from build123d import *

# Parameters (mm, degrees)
F0_R     = 1.5
F0_R_2   = 1.2
F0_R_3   = 1
F1_DEPTH = 85
F2_DEPTH = 2.5
F3_DEPTH = 4
F4_R     = 1
F6_START = -1
F5_W     = 21.3047601283
F5_H     = 75
F6_DEPTH = 1


with BuildPart() as f1:
    # F0 (on Top) → F1 (new body)
    with BuildSketch(Plane.XY):
        Circle(F0_R)
        Circle(F0_R_2, mode=Mode.SUBTRACT)
        Circle(F0_R_2)
        Circle(F0_R_3, mode=Mode.SUBTRACT)
        Circle(F0_R_3)
    extrude(amount=F1_DEPTH)

    # F0 (on Top) → F2 (cut)
    with BuildSketch(Plane.XY):
        Circle(F0_R)
        Circle(F0_R_2, mode=Mode.SUBTRACT)
    extrude(amount=F2_DEPTH, mode=Mode.SUBTRACT)

    # F0 (on Top) → F3 (cut)
    with BuildSketch(Plane.XY):
        Circle(F0_R_3)
    extrude(amount=F3_DEPTH, mode=Mode.SUBTRACT)

    # F4
    f4_edges = [f1.edges().sort_by_distance(p)[0] for p in [
        (-1.5, 0, 85),
    ]]
    fillet(f4_edges, radius=F4_R)

    # F5 (on Front) → F6 (join)
    with BuildSketch(Plane.XZ.offset(F6_START)):
        with Locations((10.6523800641, 40)):
            Rectangle(F5_W, F5_H)
    extrude(amount=-F6_DEPTH)


solid = f1.part
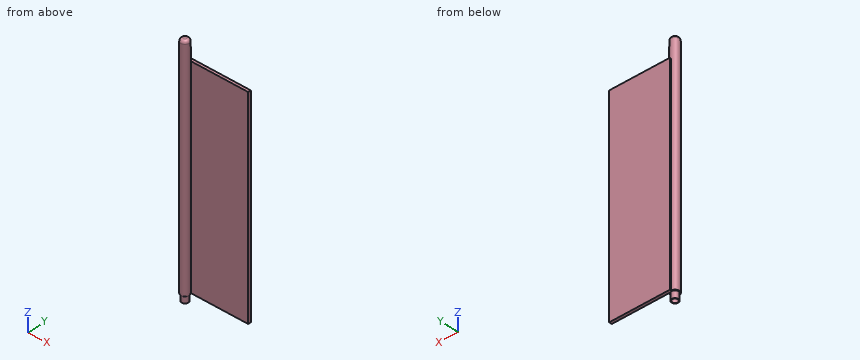
Geometry: final body of the model. Coordinates: model frame, mm. Give positions to 0.01 mm unless a question says otherwise; leave off trailing zeros. Order: outer loops, then holes, each group sorted by start corner. A loop starts at its lowest first (then second) coordinate and runs counter-clockwise, first axis right, second up. Notation, with made-up numbers: (19.25, 8.5) -> (65.25, 8.5) arc R26 cw to (65.25, 33.5) -> close; hole circle Ø7 at (-8.75, -10). An arc over 180 degrees is marked (long way). Answer as a JSON object with one key per item and string values.
Q1. First-contact query: pin 1 (0.8 mm diameter, centred on x = 6.5, y = 1.5, fed in from +Z); pin 2 (1.5 mm diameter, centred on x = 3, z = 69, fed in from -Y); pin 3 (1 mm diameter, centred on x = 9.5, y = 1, fed in from -Z); pin 4 (1 mm diameter, centred on x = 0.5, y = -0.5, fed in from -Z). Flat tips, straight axial feed; report the tip coordinate or a pass-through.
Entries:
{"pin 1": "stops at z = 77.5", "pin 2": "stops at y = 1", "pin 3": "stops at z = 2.5", "pin 4": "stops at z = 0"}
Q2. Section A-A (z = 12.5). Output: boundary loops of the cut face in (x, y), plus the area to 3 significant figures.
Entries:
{"outline": "(0, 1.5) arc R1.5 ccw (long way) to (1.12, 1) -> (21.3, 1) -> (21.3, 2) -> (0, 2) -> close", "area": "28.0 mm^2"}
Q3. Material intervals for probe 1 along Y at (x, z) = (0, 1.4); probe 2 along X at (y, z) = (-0.2, 61.5); probe 3 along Y at (x, z) = (2.25, 41.5), sorted ascending.
Entries:
{"probe 1": "y = -1.2 to -1, 1 to 1.2", "probe 2": "x = -1.49 to 1.49", "probe 3": "y = 1 to 2"}
Q4. Section B-B (x = 17.5). Output: boundary loops of the cut face in (y, z), plus the area to 3 significant figures.
Entries:
{"outline": "(1, 2.5) -> (2, 2.5) -> (2, 77.5) -> (1, 77.5) -> close", "area": "75.0 mm^2"}
